Verification items for the finished model (mm, model axes). Face numbers are marked on the shaded views. Give positions to 0.01 mm unless a question says otherwise; leave off trailing zeros. Order: outer loops, then holes, each group sorted by start corner. A loop starts at its lowest first (then second) coordinate and runs counter-clockwise, first axis right, second up.
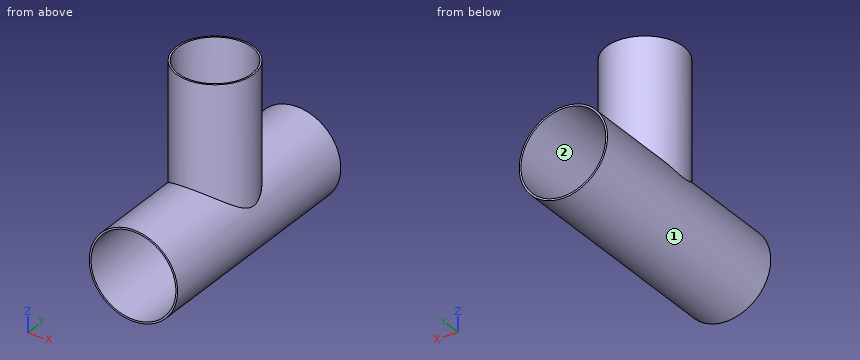
Autodesk Inventor part; units mm, degrees
ref_plane "YZ Plane" through (0, 0, 0) normal (1, 0, 0) x (0, 1, 0)
ref_plane "XZ Plane" through (0, 0, 0) normal (0, 1, 0) x (-1, 0, 0)
sketch "Sketch1" plane through (0, 0, 0) normal (0, 1, 0) x (-1, 0, 0)
  circle A0 centre (0, 0) radius 25.5
  circle A1 centre (0, 0) radius 24.5
  dimension "d0" = 51
  dimension "d1" = 49
extrude "Extrusion1" add sketch "Sketch1" along normal blind 136.878
ref_plane "Work Plane1" through (0, 0, 25.5) normal (0, 0, 1) x (1, 0, 0)
sketch "Sketch2" plane through (0, 0, 25.5) normal (0, 0, 1) x (1, 0, 0)
  line L0 (0, 0) -> (28.9243, 0) construction
  line L1 (-25.5, 0) -> (25.5, 0)
  circle A0 centre (0, 68.439) radius 21.35
  line L2 (-24.5, 136.878) -> (24.5, 136.878)
  dimension "d4" = 42.7
  dimension "d5" = 68.439
  dimension "d18" = 68.439
extrude "Extrusion2" cut sketch "Sketch2" against normal blind 25.4
sketch "Sketch3" plane through (0, 0, 25.5) normal (0, 0, 1) x (1, 0, 0)
  circle A0 centre (0, 68.439) radius 22.35
  line L0 (0, 0) -> (18.5152, 0) construction
  line L1 (24.5, 0) -> (-24.5, 0)
  circle A1 centre (0, 68.439) radius 21.35
  dimension "d8" = 68.439
  dimension "d9" = 44.7
  dimension "d10" = 42.7
extrude "Extrusion3" add sketch "Sketch3" along normal blind 60
sketch "Sketch4" plane through (0, 0, 25.5) normal (0, 0, 1) x (1, 0, 0)
  line L0 (0, 0) -> (23.949, 0) construction
  line L1 (24.5, 0) -> (-24.5, 0)
  circle A0 centre (0, 68.439) radius 22.35
  circle A1 centre (0, 68.439) radius 21.35
  dimension "d13" = 68.439
  dimension "d14" = 44.7
  dimension "d15" = 42.7
extrude "Extrusion4" add sketch "Sketch4" against normal up to next
equation "\"d5\" = d18"
equation "\"d8\" = d5"
equation "\"d10\" = d4"
equation "\"d13\" = d5"
equation "\"d15\" = d4"
properties part number "51mm nipple"
(1) Go/stop test with flat-tipped pins: pin 1 (10 mm diameter, centred on x = 8, z = 67, fed in from +Y); pin 2 (6 mm diameter, centred on x = 1, y = 81, fed in from -Z); pin 3 (12 mm diameter, centred on y = 65, z = -12.5, fed in from +X). Record where each tip stops, or that it passes through.
Solved:
pin 1: stops at y = 90.59
pin 2: stops at z = -25.5
pin 3: stops at x = 24.66
(2) Section check A-A, the plane z = 0. Enter the section's corners in (x, y), then the cut area to 3 significant figures.
Solved:
outline: (-25.5, 0) - (-24.5, 0) - (-24.5, 136.88) - (-25.5, 136.88) - close; (24.5, 0) - (25.5, 0) - (25.5, 136.88) - (24.5, 136.88) - close
area: 274 mm2
(3) Section check C-C, the plane y = 50. Enter the section's corners in (x, z).
Solved:
outline: (-12.63, 22.15) arc R25.5 ccw (long way) to (12.63, 22.15) - (12.63, 85.5) - (10.76, 85.5) - (10.76, 22.01) arc R24.5 cw (long way) to (-10.76, 22.01) - (-10.76, 85.5) - (-12.63, 85.5) - close
(4) Release check for a two-part mould opening along Z. For the marked faces 1 and 2 record: pulls with the +Z half, pulls with the -Z half, needs draft (parallel to the pull), parting line crosses it, or undercut.
Solved:
face 1: parting line crosses it
face 2: undercut
(5) Scan lines: line 1 (Y direction, x = 0, z = 45.5); line 2 (Z direction, x = -1, y = 15); line 3 (Z direction, x = -12.5, y = 121.5). Record each from-to range of solid material in increasing order.
Solved:
line 1: y = 46.09 to 47.09, 89.79 to 90.79
line 2: z = -25.48 to -24.48, 24.48 to 25.48
line 3: z = -22.23 to -21.07, 21.07 to 22.23
(6) Section check B-B, the plane x = -1.5. Enter the section's corners in (y, z).
Solved:
outline: (0, -25.46) - (136.88, -25.46) - (136.88, -24.45) - (0, -24.45) - close; (0, 24.45) - (47.14, 24.45) - (47.14, 85.5) - (46.14, 85.5) - (46.14, 25.46) - (0, 25.46) - close; (89.74, 24.45) - (136.88, 24.45) - (136.88, 25.46) - (90.74, 25.46) - (90.74, 85.5) - (89.74, 85.5) - close
(7) Section check D-D, the plane z = 74. Enter the section's corners in (x, y), then the cut area to 3 significant figures.
Solved:
outline: circle Ø44.7 at (0, 68.44); hole circle Ø42.7 at (0, 68.44)
area: 137 mm2
